Build history of the part. All positions in model axes, mm. Give positions to 0.01 mm unless a question says otherwise; leave off trailing zeros. Order: outer loops, then holes, each group sorted by start corner. A loop starts at its lowest first (then second) coordinate and runs counter-clockwise, first axis right, second up. Notation, with made-up numbers: (45, 42) - (55, 42) arc R22 cw to (55, 49) - close; hole circle Ø3 at (42.5, 6). An arc over 180 degrees is marked (long way). Write each question's results on one line, items separated by ' | '. Start each with the question number.
1) Cut at A-A on x = 0. List the corners of the cut face in (y, z).
2) Drop flat-ended pins along their axis: pin 1 Ø3 at (x, y) = (-1, 31) entering from -Z; pin 2 Ø2 at (x, z) = (0.5, 6) entering from +Y. Give the stop position or say it passes through.
3) Drill centre lines: line 1 along Z through (x, y) = (0, 44.5); line 2 along Z through (x, y) = (6.75, 15). Where is each one in solid material? Low to high. Write a range as from..to.
4) Cut at B-B on z = 0. List the corners of the cut face in (x, y).
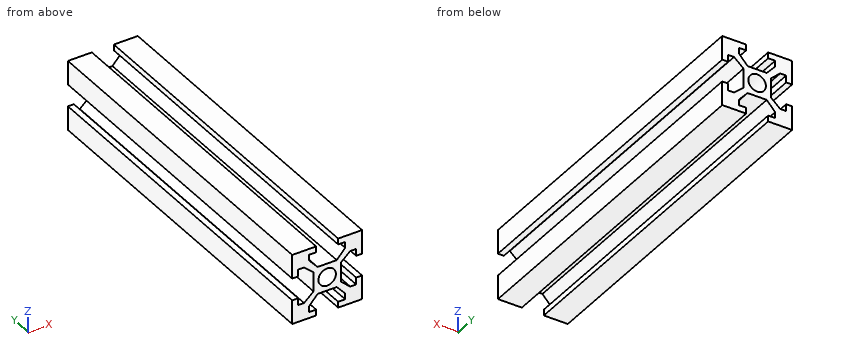
from build123d import *

# Parameters (mm, degrees)
SKETCH_1_W          = 20
SKETCH_1_H          = 20
EXTRUDE_1_DEPTH     = 100
SKETCH_2_R          = 2.5
CUT_EXTRUDE_1_DEPTH = 101


with BuildPart() as part:
    # 草图1 → 凸台-拉伸1 (new body)
    with BuildSketch(Plane(origin=(0, 0, 0), x_dir=(1, 0, 0), z_dir=(0, 1, 0))):
        Rectangle(SKETCH_1_W, SKETCH_1_H)
    extrude(amount=EXTRUDE_1_DEPTH)

    # 草图2 → 切除-拉伸1 (cut, through all)
    with BuildSketch(Plane(origin=(0, 100, 0), x_dir=(1, 0, 0), z_dir=(0, 1, 0))):
        Circle(SKETCH_2_R)
        Polygon((-3.15, 10), (-3.15, 8.3), (-5.15, 8.3), (-5.15, 6.6), (-2.75, 3.9), (2.75, 3.9), (5.15, 6.6), (5.15, 8.3), (3.15, 8.3), (3.15, 10), align=None)
        Polygon((3.9, 2.75), (3.9, -2.75), (6.6, -5.15), (8.3, -5.15), (8.3, -3.15), (10, -3.15), (10, 3.15), (8.3, 3.15), (8.3, 5.15), (6.6, 5.15), align=None)
        Polygon((2.75, -3.9), (-2.75, -3.9), (-5.15, -6.6), (-5.15, -8.3), (-3.15, -8.3), (-3.15, -10), (3.15, -10), (3.15, -8.3), (5.15, -8.3), (5.15, -6.6), align=None)
        Polygon((-3.9, -2.75), (-3.9, 2.75), (-6.6, 5.15), (-8.3, 5.15), (-8.3, 3.15), (-10, 3.15), (-10, -3.15), (-8.3, -3.15), (-8.3, -5.15), (-6.6, -5.15), align=None)
    extrude(amount=-CUT_EXTRUDE_1_DEPTH, mode=Mode.SUBTRACT)


solid = part.part
Results:
1) outline: (0, -3.9) - (100, -3.9) - (100, -2.5) - (0, -2.5) - close; (0, 2.5) - (100, 2.5) - (100, 3.9) - (0, 3.9) - close
2) pin 1: z = -3.9 | pin 2: through
3) line 1: -3.9..-2.5, 2.5..3.9 | line 2: -10..-5.15, 5.15..10
4) outline: (-3.9, 0) - (-2.5, 0) - (-2.5, 100) - (-3.9, 100) - close; (2.5, 0) - (3.9, 0) - (3.9, 100) - (2.5, 100) - close
